Autodesk Inventor part; units mm, degrees
ref_plane "part2_to_part1_XY" through (0, 0, 0) normal (1, 0, 0) x (0, 0, -1)
ref_plane "part2_to_part1_YZ" through (0, 0, 0) normal (0, 0, -1) x (0, 1, 0)
ref_plane "part2_to_part1_ZX" through (0, 0, 0) normal (0, 1, 0) x (1, 0, 0)
sketch "Sketch_1" plane through (0, 0, 0) normal (0, 0, 1) x (1, 0, 0)
  line L0 (6, 0) -> (0, 0)
  line L1 (1, 4) -> (6, 4)
  line L2 (6, 4) -> (6, 9.5)
  line L3 (6, 9.5) -> (5.5, 10)
  line L4 (5.5, 10) -> (1, 10)
  line L5 (1, 10) -> (1, 4)
revolve "Revolution1" add sketch "Sketch_1" angle 180 mid plane about axis through (6, 0, 0) along (-1, 0, 0)
sketch "Sketch_2" plane through (0, 0, 0) normal (0, 0, 1) x (1, 0, 0)
  line L0 (0, 0.5) -> (0, 0)
  line L1 (0, 0) -> (16, 0)
  line L2 (16, 0) -> (16, 0.5)
  line L3 (16, 0.5) -> (0, 0.5)
extrude "Extrusion1" cut sketch "Sketch_2" along normal mid plane 40
sketch "Sketch_3" plane through (0, 0, 7) normal (0, 0, 1) x (1, 0, 0)
  line L0 (3.5, 10) -> (3.5, 0)
  line L1 (3.5, 0) -> (1.75, 0)
  line L2 (1.75, 0) -> (1.75, 3.5)
  line L3 (1.75, 3.5) -> (0.25, 3.5)
  line L4 (0.25, 3.5) -> (0.25, 10)
  line L5 (0.25, 10) -> (3.5, 10)
  line L6 (3.5, 10) -> (3.5, 0)
sketch "Sketch_4" plane through (0, 0, -7) normal (0, 0, 1) x (1, 0, 0)
  line L0 (3.5, 10) -> (3.5, 0)
  line L1 (3.5, 0) -> (1.75, 0)
  line L2 (1.75, 0) -> (1.75, 3.5)
  line L3 (1.75, 3.5) -> (0.25, 3.5)
  line L4 (0.25, 3.5) -> (0.25, 10)
  line L5 (0.25, 10) -> (3.5, 10)
  line L6 (3.5, 10) -> (3.5, 0)
ref_plane "part2_to_part1_XY" through (0, 0, 0) normal (1, 0, 0) x (0, 0, -1)
ref_plane "part2_to_part1_YZ" through (0, 0, 0) normal (0, 0, -1) x (0, 1, 0)
ref_plane "part2_to_part1_ZX" through (0, 0, 0) normal (0, 1, 0) x (1, 0, 0)
ref_plane "part2_to_screw1_XY" through (3.5, 3.5, 7) normal (0, 1, 0) x (1, 0, 0)
ref_plane "part2_to_screw1_YZ" through (3.5, 3.5, 7) normal (1, 0, 0) x (0, 0, -1)
ref_plane "part2_to_screw1_ZX" through (3.5, 3.5, 7) normal (0, 0, -1) x (0, 1, 0)
ref_plane "part2_to_screw2_XY" through (3.5, 3.5, -7) normal (0, 1, 0) x (1, 0, 0)
ref_plane "part2_to_screw2_YZ" through (3.5, 3.5, -7) normal (1, 0, 0) x (0, 0, -1)
ref_plane "part2_to_screw2_ZX" through (3.5, 3.5, -7) normal (0, 0, -1) x (0, 1, 0)
sketch "スケッチ7" plane through (6, 0, 0) normal (1, 0, 0) x (0, 0, -1)
  circle A0 centre (0, 0) radius 5.1
  dimension "d11" = 10.2
extrude "押し出し4" cut sketch "スケッチ7" against normal blind 10
ref_plane "作業平面10" through (3.25, 10, 0) normal (0, 1, 0) x (-1, 0, 0)
sketch "スケッチ8" plane through (3.25, 10, 0) normal (0, 1, 0) x (-1, 0, 0)
  circle A0 centre (-0.25, 7) radius 1.75
  circle A1 centre (-0.25, 7) radius 1.7
  circle A2 centre (-0.25, 7) radius 3.5
  circle A3 centre (-0.25, -7) radius 1.75
  circle A4 centre (-0.25, -7) radius 1.7
  circle A5 centre (-0.25, -7) radius 3.5
  point P0 (3.25, 0)
  dimension "d14" = 3.4
  dimension "d15" = 7
  dimension "d16" = 3.4
  dimension "d17" = 7
extrude "押し出し5" cut sketch "スケッチ8" against normal through all contours A1 | A4
extrude "押し出し6" cut sketch "スケッチ8" against normal blind 5 contours A0 | A1 | A2 | A3 | A4 | A5
properties part number "MBRDAC23-2-8_p2"
For this review, take the finished solid that the model builds, in its own axes (mm). A direction names the side the tool comes from. Give positions to 0.01 mm unless a question says otherwise; leave off trailing zeros. Order: outer loops, then holes, each group sorted by start corner. A loop starts at its lowest first (then second) coordinate and runs counter-clockwise, first axis right, second up. Notation, with made-up numbers: M 50.5,-27.75 L 80.5,-27.75 A24 ccw 80.5,3.25 Z; hole C 36.25,68.25 d3. An arc over 180 degrees is marked long. Answer in a Markdown table with one row per item. Add a question column.
(1) For pin 1 (5 mm diameter, centred on y = 6, z = 5.5, fed in from -X); pin 2 (2 mm diameter, centred on x = 3.5, z = -7, fed in from -Y) (3 decimals), all flat-tipped, find the tip position at first contact; note any pin that passes through.
(2) Consider section A-A on z = 7. State the section outline as (x, y) points, and give its area (3 significant figures).
(3) Consider section D-D on z = -5.75. State the section outline as (x, y) points, and give its area (3 significant figures).
(4) For faces 5 (the face through (5.86, 9.64, 0.07)), 6 (the face through (3.5, 7.2, -3.5)), 7 (the face through (4, 5, 5)), list the 3-axis set-ups (+Z, -Z, +X, -X, +Y, -Y) from which the entire face can be reached by the end or side of a thin tool; tool diameter is ignored.
(5) Wall thickness on probe 1 along X at (y, z) = (2.2, 7); probe 2 along Z at (x, y) = (3.5, 2.3); probe 3 along Z at (x, y) = (2.85, 3.75): over which ranges is each line inside the solid? List them lowest first. Write a range as [from, to].
(6) Consider section B-B on x = 3.5. State the section outline as (y, z) points.
(7) Mouldability with a two-part tool opening along X and no side actions: class faces 1 (the face through (3.5, 7.2, 3.5)), 2 (the face through (5, 0.5, 9)), 3 (the face through (5.8, 2.92, -9.25)), 4 (the face through (2.7, 2.8, -8.5)) as +X half, -X half, draft (parallel to the pull), parting line (faces both ways), or undercut.
(8) Consider section C-C on y = 2. Give the number of separate pieces and of enclosed holes in the cut face, and give its area (3 significant figures).
Evaluation:
| question | item | result |
|---|---|---|
| 1 | pin 1 | stops at x = 1 |
| 1 | pin 2 | passes through |
| 2 | outline | M 1,0.5 L 1.8,0.5 L 1.8,5 L 1,5 Z; M 5.2,0.5 L 6,0.5 L 6,5 L 5.2,5 Z |
| 2 | area | 7.20 mm^2 |
| 3 | outline | M 1,0.5 L 2.35,0.5 L 2.35,5 L 1,5 Z; M 4.65,0.5 L 6,0.5 L 6,5 L 4.65,5 Z |
| 3 | area | 12.1 mm^2 |
| 4 | face 5 | +X, +Y |
| 4 | face 6 | -Z, +Y |
| 4 | face 7 | +Z, +Y |
| 5 | probe 1 | x = [1, 1.8], [5.2, 6] |
| 5 | probe 2 | z = [-9.73, -8.7], [-5.3, -4.55], [4.55, 5.3], [8.7, 9.73] |
| 5 | probe 3 | z = [-9.27, -8.57], [-5.43, -3.46], [3.46, 5.43], [8.57, 9.27] |
| 6 | outline | M 0.5,-9.99 A10 ccw 4.93,-8.7 L 0.5,-8.7 Z; M 0.5,-5.3 L 5,-5.3 L 5,-3.5 L 9.37,-3.5 A10 ccw 9.37,3.5 L 5,3.5 L 5,5.3 L 0.5,5.3 L 0.5,5.08 A5.1 cw 0.5,-5.08 Z; M 0.5,8.7 L 4.93,8.7 A10 ccw 0.5,9.99 Z |
| 7 | face 1 | undercut |
| 7 | face 2 | draft |
| 7 | face 3 | +X half |
| 7 | face 4 | undercut |
| 8 | separate pieces | 2 |
| 8 | enclosed holes | 2 |
| 8 | area | 32.7 mm^2 |
